```python
from build123d import *

# Parameters (mm, degrees)
BOSS_EXTRUDE1_DEPTH = 22
SKETCH2_R           = 1.5
CUT_EXTRUDE1_DEPTH  = 3
SKETCH3_R           = 6.62
SKETCH3_R_2         = 4.5
BOSS_EXTRUDE2_DEPTH = 1
SKETCH3_3_R         = 3
BOSS_EXTRUDE3_DEPTH = 16
SKETCH4_R           = 12
BOSS_EXTRUDE4_DEPTH = 39


with BuildPart() as part:
    # Sketch1 → Boss-Extrude1 (new body)
    with BuildSketch(Plane.XY):
        with BuildLine():
            Line((-21, -16), (21, -16))
            ThreePointArc((21, -16), (22.414213562, -15.414213562), (23, -14))
            Line((23, -14), (23, 14))
            ThreePointArc((23, 14), (22.414213562, 15.414213562), (21, 16))
            Line((21, 16), (-21, 16))
            ThreePointArc((-21, 16), (-22.414213562, 15.414213562), (-23, 14))
            Line((-23, 14), (-23, -14))
            ThreePointArc((-23, -14), (-22.414213562, -15.414213562), (-21, -16))
        make_face()
    extrude(amount=BOSS_EXTRUDE1_DEPTH)

    # Sketch2 → Cut-Extrude1 (cut)
    with BuildSketch(Plane.XY.offset(22)):
        with Locations((-16.45, 9.1)):
            Circle(SKETCH2_R)
        with Locations((16.45, 9.1)):
            Circle(SKETCH2_R)
        with Locations((16.4, -9.099931319)):
            Circle(SKETCH2_R)
        with Locations((-16.5, -9.099931319)):
            Circle(SKETCH2_R)
    extrude(amount=-CUT_EXTRUDE1_DEPTH, mode=Mode.SUBTRACT)

    # Sketch3 → Boss-Extrude2 (add)
    with BuildSketch(Plane.XY.offset(22)):
        with Locations((-8.2, 0)):
            Circle(SKETCH3_R)
        with Locations((-8.2, 0)):
            Circle(SKETCH3_R_2, mode=Mode.SUBTRACT)
    extrude(amount=BOSS_EXTRUDE2_DEPTH)

    # Sketch3<3> → Boss-Extrude3 (add)
    with BuildSketch(Plane.XY.offset(22)):
        with Locations((-8.2, 0)):
            Circle(SKETCH3_3_R)
    extrude(amount=BOSS_EXTRUDE3_DEPTH)

    # Sketch4 → Boss-Extrude4 (add)
    with BuildSketch(Plane(origin=(23, 0, 0), x_dir=(0, 0, -1), z_dir=(1, 0, 0))):
        with Locations((-10, 0)):
            Circle(SKETCH4_R)
    extrude(amount=BOSS_EXTRUDE4_DEPTH)


solid = part.part
```
The model under review builds one solid part; all positions refer to its coordinate system, in mm. A direction names the side the tool comes from. Give positions to 0.01 mm unless a question says otherwise; leave off trailing zeros. Write each loop counter-clockwise with the first axis right and the second up, starting at its lowest first coordinate (ties: lowest second). Pieces come first, ordered by that corner, then holes. Notation, with made-up numbers: (7.25, 47.25) -> (48.25, 47.25) arc R15 cw to (48.25, 76.25) -> close; hole circle Ø5 at (83.25, 79). An arc over 180 degrees is marked (long way). Put each result on its own line as item: value.
(1) We need section B-B, the plane z = 20. Give the boundary of the cut face in (x, y), and give its area (3 significant figures).
Results are:
outline: (-23, -14) arc R2 ccw to (-21, -16) -> (21, -16) arc R2 ccw to (23, -14) -> (23, -6.63) -> (62, -6.63) -> (62, 6.63) -> (23, 6.63) -> (23, 14) arc R2 ccw to (21, 16) -> (-21, 16) arc R2 ccw to (-23, 14) -> close; hole circle Ø3 at (-16.5, -9.1); hole circle Ø3 at (-16.45, 9.1); hole circle Ø3 at (16.4, -9.1); hole circle Ø3 at (16.45, 9.1)
area: 1,960 mm²
(2) We need section C-C, the plane z = 8. Give the boundary of the cut face in (x, y).
Results are:
outline: (-23, -14) arc R2 ccw to (-21, -16) -> (21, -16) arc R2 ccw to (23, -14) -> (23, -11.83) -> (62, -11.83) -> (62, 11.83) -> (23, 11.83) -> (23, 14) arc R2 ccw to (21, 16) -> (-21, 16) arc R2 ccw to (-23, 14) -> close
(3) For pin 1 Ø2.5 at (x, y) = (16.4, -9.1) entering from -Z; pin 2 Ø3.5 at (x, y) = (-16, 9.5) entering from +Z; pin 3 Ø3 at (x, y) = (44.5, -5) entering from +Z, all flat-tipped, find the tip position at first contact; note any pin that passes through.
Results are:
pin 1: z = 0
pin 2: z = 22
pin 3: z = 21.48
(4) We need section D-D, the plane y = 2. Give the boundary of the cut face in (x, z), and give its area (3 significant figures).
Results are:
outline: (-23, 0) -> (23, 0) -> (23, -1.83) -> (62, -1.83) -> (62, 21.83) -> (23, 21.83) -> (23, 22) -> (-1.89, 22) -> (-1.89, 23) -> (-4.17, 23) -> (-4.17, 22) -> (-5.96, 22) -> (-5.96, 38) -> (-10.44, 38) -> (-10.44, 22) -> (-12.23, 22) -> (-12.23, 23) -> (-14.51, 23) -> (-14.51, 22) -> (-23, 22) -> close
area: 2,010 mm²
(5) We need section A-A, the plane x = -8.2. Give the boundary of the cut face in (y, z), and give its area (3 significant figures).
Results are:
outline: (-16, 0) -> (16, 0) -> (16, 22) -> (6.62, 22) -> (6.62, 23) -> (4.5, 23) -> (4.5, 22) -> (3, 22) -> (3, 38) -> (-3, 38) -> (-3, 22) -> (-4.5, 22) -> (-4.5, 23) -> (-6.62, 23) -> (-6.62, 22) -> (-16, 22) -> close
area: 804 mm²
(6) To check wall thickness, follow probe 1 along Y at (x, z) = (-16.45, 21.3); probe 2 along Z at (x, y) = (6.5, -6); probe 3 along Y at (x, z) = (-16, 20). State the ranges of each line that lie inside material, in increasing order. Write a range as from..to.
Results are:
probe 1: -16..-10.6, -7.6..7.6, 10.6..16
probe 2: 0..22
probe 3: -16..-10.51, -7.69..7.67, 10.53..16
(7) Tool access review of faces 1 (the flat face through (23, 12, 13)), 2 (the flat face through (23, -12, 12)), 3 (the flat face through (23, 0, -1)), 4 (the cylindrical face through (42.227, -7.302, 19.523)), 5 (the flat face through (-16, 9, 19)): name each direction out of +Z, -Z, +X, -X, +Y, -Y from which nothing blocks a thin tool from reaching the whole face with its end or side.
Results are:
face 1: +X, +Y
face 2: +X, -Y
face 3: -Z, -X, +Y, -Y
face 4: +X
face 5: +Z
